Input: part model. Units: mm. Frame: model coordinates. Coordinates: 2 decimals unless noted, no trailing zeros. Order: outer loops, then holes, each group sorted by start corner. A loop starts at its lowest first (then second) coordinate and runs counter-clockwise, first axis right, second up. Notation, with made-up numbers: (-7.5, -29.5) -> (36.5, -29.5) arc R23 cw to (36.5, -17.5) -> close; hole circle Ø9 at (85, 37.5). An arc over 180 degrees is marked (long way). Write each question's results on one line, items separated by ' | '.
```python
from build123d import *

# Parameters (mm, degrees)
BOSS_EXTRUDE1_DEPTH     = 12.7
SKETCH2_W               = 19.216952518
SKETCH2_H               = 6.005297662
CUT_EXTRUDE1_DEPTH      = 2.54
SKETCH3_W               = 18.322345719
SKETCH3_H               = 4.189551825
SKETCH3_R               = 1.155216028
CUT_EXTRUDE2_DEPTH      = 11.684
CUT_EXTRUDE2_DEPTH_BACK = 26.924
SKETCH4_W               = 6.230536122
SKETCH4_H               = 1.706386664
SKETCH4_W_2             = 6.230536121
SKETCH4_H_2             = 1.682353049
CUT_EXTRUDE4_DEPTH      = 3.81
SKETCH5_W               = 12.461072243
SKETCH5_H               = 1.883415491
CUT_EXTRUDE5_DEPTH      = 2.54
SKETCH6_W               = 6.43751361
SKETCH6_H               = 1.686706137
SKETCH6_H_2             = 1.657293844
CUT_EXTRUDE6_DEPTH      = 1.0000001
CUT_EXTRUDE6_DEPTH_BACK = 3.81


with BuildPart() as part:
    # Sketch1 → Boss-Extrude1 (new body)
    with BuildSketch(Plane(origin=(0, 0, 0), x_dir=(1, 0, 0), z_dir=(0, 1, 0))):
        with BuildLine():
            Line((0, 0), (19.216952518, 0))
            Line((19.216952518, 0), (19.216952518, 6.005297662))
            Line((19.216952518, 6.005297662), (26.423309712, 6.005297662))
            add(Edge.make_bspline(
                [(26.423309712, 6.005297662), (36.55952446, 42.663140535), (-2.021004002, 14.397041287), (-6.085368297, 6.005297662)],
                knots=[0, 0, 0, 0, 1, 1, 1, 1], degree=3))
            Line((-6.085368297, 6.005297662), (0, 6.005297662))
            Line((0, 6.005297662), (0, 0))
        make_face()
    extrude(amount=BOSS_EXTRUDE1_DEPTH)

    # Sketch2 → Cut-Extrude1 (cut)
    with BuildSketch(Plane(origin=(0, 12.7, 0), x_dir=(1, 0, 0), z_dir=(0, 1, 0))):
        with Locations((9.608476259, 3.002648831)):
            Rectangle(SKETCH2_W, SKETCH2_H)
    extrude(amount=-CUT_EXTRUDE1_DEPTH, mode=Mode.SUBTRACT)

    # Sketch3 → Cut-Extrude2 (cut, two sides)
    with BuildSketch(Plane(origin=(19.216952518, 0, 0), x_dir=(0, 0, -1), z_dir=(1, 0, 0))) as cut_extrude2_sk:
        Polygon((24.327643381, 12.7), (6.005297662, 12.7), (24.327643381, 4.189551825), align=None)
        with Locations((15.166470522, 2.094775913)):
            Rectangle(SKETCH3_W, SKETCH3_H)
        Polygon((3.002648831, 4.189551825), (0, 4.189551825), (0, 0), (6.005297662, 0), (6.005297662, 4.189551825), align=None)
        with BuildLine():
            Line((3.002648831, 10.16), (0, 10.16))
            Line((0, 10.16), (0, 4.189551825))
            Line((0, 4.189551825), (3.002648831, 4.189551825))
            ThreePointArc((3.002648831, 4.189551825), (0.017424743, 7.174775912), (3.002648831, 10.16))
        make_face()
        with Locations((3.002648831, 7.174775912)):
            Circle(SKETCH3_R)
    extrude(amount=CUT_EXTRUDE2_DEPTH, mode=Mode.SUBTRACT)
    extrude(cut_extrude2_sk.sketch, amount=-CUT_EXTRUDE2_DEPTH_BACK, mode=Mode.SUBTRACT)

    # Sketch4 → Cut-Extrude4 (cut)
    with BuildSketch(Plane(origin=(0, 12.740629014, -5.917826495), x_dir=(1, 0, 0), z_dir=(0, 0.906940046, -0.421259722))):
        with Locations((6.493208198, 8.028748928)):
            Rectangle(SKETCH4_W, SKETCH4_H)
        with Locations((12.72374432, 8.028748928)):
            Rectangle(SKETCH4_W_2, SKETCH4_H)
        with Locations((12.72374432, 4.676059638)):
            Rectangle(SKETCH4_W_2, SKETCH4_H_2)
        with Locations((6.493208198, 4.676059638)):
            Rectangle(SKETCH4_W, SKETCH4_H_2)
    extrude(amount=-CUT_EXTRUDE4_DEPTH, mode=Mode.SUBTRACT)

    # Sketch5 → Cut-Extrude5 (cut)
    with BuildSketch(Plane(origin=(0, -2.32418937, -5.003802419), x_dir=(1, 0, 0), z_dir=(0, 0.421259722, 0.906940046))):
        with Locations((9.608476259, 11.179636351)):
            Rectangle(SKETCH5_W, SKETCH5_H)
    extrude(amount=-CUT_EXTRUDE5_DEPTH, mode=Mode.SUBTRACT)

    # Sketch6 → Cut-Extrude6 (cut, two sides)
    with BuildSketch(Plane(origin=(0, 4.189551825, 0), x_dir=(-1, 0, 0), z_dir=(0, -1, 0))) as cut_extrude6_sk:
        with Locations((-6.389719454, 9.230258043)):
            Rectangle(SKETCH6_W, SKETCH6_H)
        with Locations((-12.827233064, 9.230258043)):
            Rectangle(SKETCH6_W, SKETCH6_H)
        with Locations((-12.827233064, 12.681510307)):
            Rectangle(SKETCH6_W, SKETCH6_H_2)
        with Locations((-6.389719454, 12.681510307)):
            Rectangle(SKETCH6_W, SKETCH6_H_2)
    extrude(amount=CUT_EXTRUDE6_DEPTH, mode=Mode.SUBTRACT)
    extrude(cut_extrude6_sk.sketch, amount=-CUT_EXTRUDE6_DEPTH_BACK, mode=Mode.SUBTRACT)


solid = part.part
```
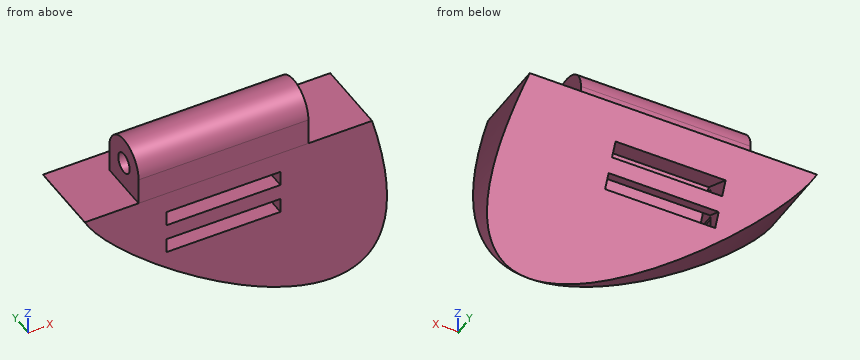
(1) Pin query (flat end, axial travel): P1, Ø3, axis at x = 7.5, z = -20, coming from the +Y side; P2, Ø1.9, axis at y = 7, z = -9, coming from the +X side; P3, Ø2.5, axis at y = 8.5, z = -11, coming from the +X side; P4, Ø1.8, axis at y = 7.17, z = -3, coming from the -X side. Return the tip coordinate at first contact, or that it passes through.
Return value:
P1: y = 6.9 | P2: x = 27.38 | P3: x = 27.79 | P4: through
(2) Line query: line 1 along X through (y, z) = (5.25, -1); line 2 along Y through (x, z) = (13, -4); line 3 along Z through (x, y) = (6, 7.75). Output: solid intervals per line, ascending. Write a range as from..to.
Return value:
line 1: 0..19.22 | line 2: 4.19..6.59, 7.76..10.16 | line 3: -16.66..-13.51, -7.83..-4, -2..-0.07
(3) Cut plane A-A, the plane z = -2.5. Return loops of the section in (x, y).
Return value:
outline: (0, 4.23) -> (19.22, 4.23) -> (19.22, 6.13) -> (0, 6.13) -> close; (0, 8.21) -> (19.22, 8.21) -> (19.22, 10.12) -> (0, 10.12) -> close
(4) Cut plane B-B, the plane x = 12.5. Count the separate pieces of the cut face and the enclosed holes in it, plus the area to 3 significant figures.
Return value:
separate pieces: 4 | enclosed holes: 1 | area: 79.4 mm2
(5) Cut plane C-C, the plane z = -5. Return loops of the section in (x, y), plus the area to 3 significant figures.
Return value:
outline: (0, 4.19) -> (19.22, 4.19) -> (19.22, 10.16) -> (0, 10.16) -> close | area: 115 mm2
